```python
from build123d import *

# Parameters (mm, degrees)
SKETCH1_W           = 101
SKETCH1_H           = 40
SKETCH1_R           = 11
SKETCH1_R_2         = 10
BOSS_EXTRUDE1_DEPTH = 30
FILLET1_R           = 30
FILLET2_R           = 30
BOSS_EXTRUDE2_DEPTH = 12.7
LPATTERN2_COUNT     = 2
LPATTERN2_PITCH     = 427.3
CUT_EXTRUDE1_REACH  = 295.353
SKETCH3_R           = 15


with BuildPart() as part:
    # Sketch1 → Boss-Extrude1 (new body)
    # profile 1 of 3: a face of its own
    with BuildSketch(Plane(origin=(0, 0, 0), x_dir=(1, 0, 0), z_dir=(0, 1, 0))):
        with Locations((-124.5, -30)):
            Rectangle(SKETCH1_W, SKETCH1_H)
        with Locations(Location((-145, -30, 0), (0, 0, 270))):
            Circle(SKETCH1_R, mode=Mode.SUBTRACT)
        with Locations(Location((-104, -30, 0), (0, 0, 270))):
            Circle(SKETCH1_R_2, mode=Mode.SUBTRACT)
    # profile 2 of 3: a face of its own
    with BuildSketch(Plane(origin=(0, 0, 0), x_dir=(1, 0, 0), z_dir=(0, 1, 0))):
        Polygon((220, 10), (-220, 10), (-220, -10), (-217.730894996, -10), (-215.497523929, -10), (-204.607421626, -10), (-182.730894996, -10), (-175, -10), (-74, -10), (74, -10), (175, -10), (220, -10), align=None)
    # profile 3 of 3: a face of its own
    with BuildSketch(Plane(origin=(0, 0, 0), x_dir=(1, 0, 0), z_dir=(0, 1, 0))):
        with Locations((124.5, -30)):
            Rectangle(SKETCH1_W, SKETCH1_H)
        with Locations(Location((104, -30, 0), (0, 0, 270))):
            Circle(SKETCH1_R_2, mode=Mode.SUBTRACT)
        with Locations(Location((145, -30, 0), (0, 0, 270))):
            Circle(SKETCH1_R, mode=Mode.SUBTRACT)
    extrude(amount=BOSS_EXTRUDE1_DEPTH)

    # Fillet1
    fillet1_edges = [part.edges().sort_by_distance(p)[0] for p in [
        (-74, 15, 10),
    ]]
    fillet(fillet1_edges, radius=FILLET1_R)

    # Fillet2
    fillet2_edges = [part.edges().sort_by_distance(p)[0] for p in [
        (74, 15, 10),
    ]]
    fillet(fillet2_edges, radius=FILLET2_R)

    # Sketch2 → Boss-Extrude2 (add)
    with BuildSketch(Plane(origin=(220, 0, 0), x_dir=(0, 0, -1), z_dir=(1, 0, 0))):
        with BuildLine():
            Line((20.00915922, 34.992960702), (-15.016204221, 34.992960702))
            ThreePointArc((-15.016204221, 34.992960702), (-18.550303731, 33.529088755), (-20.014175678, 29.994989245))
            Line((-20.014175678, 29.994989245), (-20.014175678, -1.642e-06))
            ThreePointArc((-20.014175678, -1.642e-06), (-18.550303731, -3.534101152), (-15.016204221, -4.997973099))
            Line((-15.016204221, -4.997973099), (20.019193394, -4.997973099))
            Line((20.019193394, -4.997973099), (132.5, -20))
            Line((132.5, -20), (182.5, -20))
            ThreePointArc((182.5, -20), (186.035533906, -18.535533906), (187.5, -15))
            Line((187.5, -15), (187.5, 45))
            ThreePointArc((187.5, 45), (186.035533906, 48.535533906), (182.5, 50))
            Line((182.5, 50), (132.5, 50))
            Line((132.5, 50), (20.00915922, 34.992960702))
        make_face()
    boss_extrude2 = extrude(amount=-BOSS_EXTRUDE2_DEPTH)

    # LPattern2: Boss-Extrude2 ×2
    with Locations(*[(-i * LPATTERN2_PITCH, 0, 0) for i in range(1, LPATTERN2_COUNT)]):
        add(boss_extrude2)

    # Sketch3 → Cut-Extrude1 (cut, up to next)
    with BuildSketch(Plane(origin=(0, 30, 0), x_dir=(1, 0, 0), z_dir=(0, 1, 0)), mode=Mode.PRIVATE) as cut_extrude1_sk1:
        with Locations(Location((-104, -30, 0), (0, 0, 270))):
            Circle(SKETCH3_R)
    cut_extrude1_tool1 = extrude(cut_extrude1_sk1.sketch, amount=-CUT_EXTRUDE1_REACH, mode=Mode.PRIVATE) & part.part
    # Sketch3 → Cut-Extrude1 (cut, up to next)
    with BuildSketch(Plane(origin=(0, 30, 0), x_dir=(1, 0, 0), z_dir=(0, 1, 0)), mode=Mode.PRIVATE) as cut_extrude1_sk2:
        with Locations(Location((104, -30, 0), (0, 0, 270))):
            Circle(SKETCH3_R)
    cut_extrude1_tool2 = extrude(cut_extrude1_sk2.sketch, amount=-CUT_EXTRUDE1_REACH, mode=Mode.PRIVATE) & part.part
    add(cut_extrude1_tool1.solids().sort_by_distance((-104, 30, 30))[0], mode=Mode.SUBTRACT)
    add(cut_extrude1_tool2.solids().sort_by_distance((104, 30, 30))[0], mode=Mode.SUBTRACT)


solid = part.part
```
The model under review builds one solid part; all positions refer to its coordinate system, in mm. A direction names the side the tool comes from. Round coordinates to 2 decimals unless told otherwise and drop trailing zeros. Order: outer loops, then holes, each group sorted by start corner. A loop starts at its lowest first (then second) coordinate and runs counter-clockwise, first axis right, second up. Notation, with made-up numbers: (-38, 28) -> (-4, 28) arc R21 cw to (-4, 63) -> close; hole circle Ø1 at (30.5, -17). An arc over 180 degrees is marked (long way). Use a Markdown table: item, result.
Q1. We need section B-B on y = 21.5. Write out the cut boundary in (x, z).
Values:
| item | result |
|---|---|
| outline | (-220, -187.5) -> (-207.3, -187.5) -> (-207.3, -10) -> (207.3, -10) -> (207.3, -187.5) -> (220, -187.5) -> (220, 20.01) -> (207.3, 20.01) -> (207.3, 10) -> (175, 10) -> (175, 50) -> (74, 50) -> (74, 40) arc R30 cw to (44, 10) -> (-44, 10) arc R30 cw to (-74, 40) -> (-74, 50) -> (-175, 50) -> (-175, 10) -> (-207.3, 10) -> (-207.3, 20.01) -> (-220, 20.01) -> close; hole circle Ø22 at (-145, 30); hole circle Ø30 at (-104, 30); hole circle Ø30 at (104, 30); hole circle Ø22 at (145, 30) |
Q2. We need section D-D on x = -191.5. Write out the cut boundary in (y, z).
Values:
| item | result |
|---|---|
| outline | (0, -10) -> (30, -10) -> (30, 10) -> (0, 10) -> close |
Q3. Clearance check with flat-ended pins moving along their axes: P1, Ø9, axis at x = 24.5, y = 17, coming from the -Z side; P2, Ø3, axis at y = 16, z = 42.5, coming from the -X side; P3, Ø15, axis at x = -185.5, y = 11.5, coming from the +Z side; P4, Ø8, axis at x = -112, y = -7.5, coming from the -Z side. State where each tip first meets the part, or that it passes through.
Values:
| item | result |
|---|---|
| P1 | stops at z = -10 |
| P2 | stops at x = -175 |
| P3 | stops at z = 10 |
| P4 | passes through |
Q4. For line 1 (Z direction, x = -105, y = 13); line 2 (X direction, y = -0.5, z = -174.5); line 3 (X direction, y = 23, z = 36), list the stretches that pass through material, from the lowest coordinate up.
Values:
| item | result |
|---|---|
| line 1 | z = -10 to 15.03, 44.97 to 50 |
| line 2 | x = -220 to -207.3, 207.3 to 220 |
| line 3 | x = -175 to -154.22, -135.78 to -117.75, -90.25 to -73.73, 73.73 to 90.25, 117.75 to 135.78, 154.22 to 175 |
Q5. Mouldability with a two-part tool opening along X and no side actions: class faces 1 (the flat face through (-3, 0, 6)), 2 (the flat face through (213.74, 42.6, -77.04)) as +X half, -X half, draft (parallel to the pull), parting line (faces both ways), or undercut.
Values:
| item | result |
|---|---|
| face 1 | undercut |
| face 2 | draft |
Q6. Tool access review of faces 3 (the flat face through (214, 34.993, -3)), 4 (the flat face through (214, 15, 20.014)), 5 (the cylindrical face through (64.979, 15.21, 18.555)): name each direction out of +Z, -Z, +X, -X, +Y, -Y from which nothing blocks a thin tool from reaching the whole face with its end or side.
Values:
| item | result |
|---|---|
| face 3 | +Z, +X, -X, +Y |
| face 4 | +Z, +X, +Y, -Y |
| face 5 | +Z, +Y, -Y |
Q7. We need section C-C on z = -162.5. Write out the cut boundary in (x, y), then the cut area to 3 significant figures.
Values:
| item | result |
|---|---|
| outline | (-220, -20) -> (-207.3, -20) -> (-207.3, 50) -> (-220, 50) -> close; (207.3, -20) -> (220, -20) -> (220, 50) -> (207.3, 50) -> close |
| area | 1,780 mm^2 |
Q8. We need section A-A on x = 104. Write out the cut boundary in (y, z), then the cut area to 3 significant figures.
Values:
| item | result |
|---|---|
| outline | (0, -10) -> (30, -10) -> (30, 15) -> (0, 15) -> close; (0, 45) -> (30, 45) -> (30, 50) -> (0, 50) -> close |
| area | 900 mm^2 |
